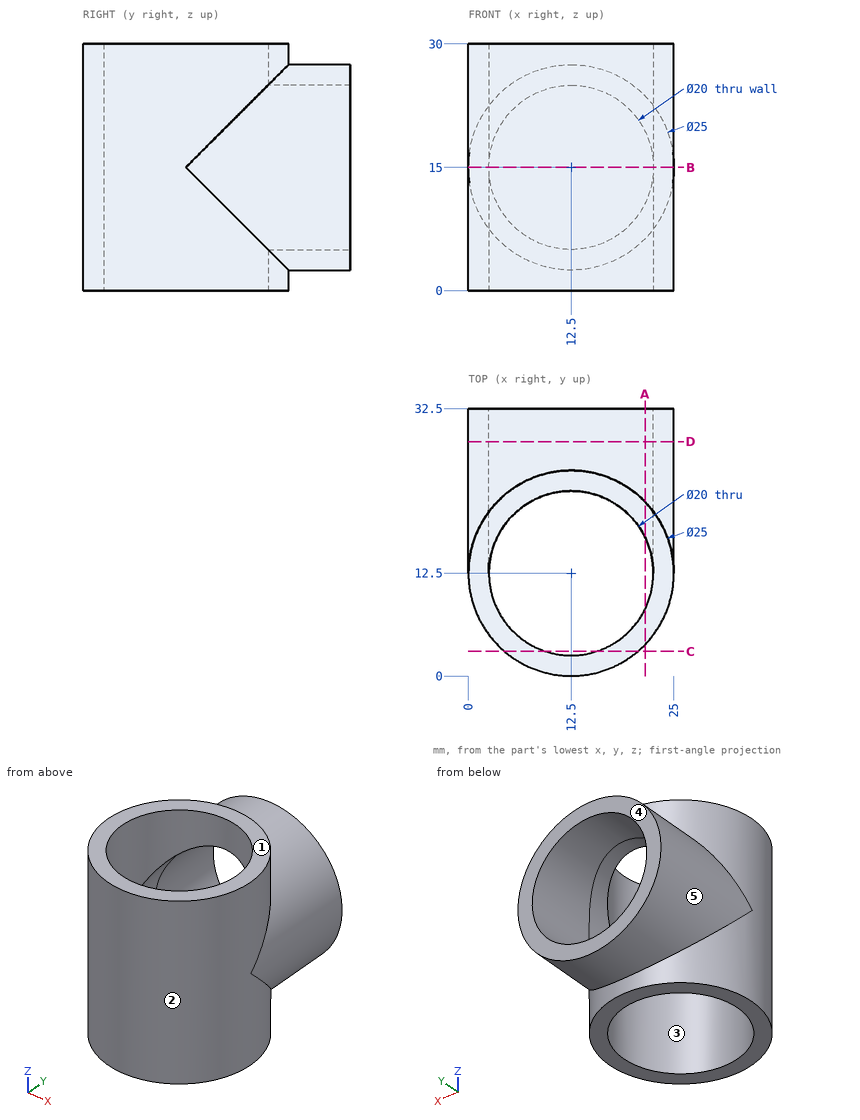
Study the drawing (mm; zero at the part's minimum x, y, z) and answer. A direction names the side the tool comes from. Give positions to 0.01 mm unless a question says otherwise; leave off trailing zeros. Loops run counter-clockwise (first coordinate to the right, second up) from the corner with the lowest first, then second, coordinate; pieces in that order, holes last. Notation, with made-up numbers: M 76.5,13.25 L 85.5,13.25 A28 ccw 85.5,38.25 Z; hole C -7,4 d9. An arc over 180 degrees is marked long. One line per item, written item: value.
1. Section D-D on y = 28.5 is taken. Determine the outline of the cut face in (x, z), plus the area to 3 significant figures.
Found:
outline: C 12.5,15 d25; hole C 12.5,15 d20
area: 177 mm^2
2. Find the intervals of material crossed by probe 1 along X at (y, z) = (12.5, 6.5); probe 2 along Y at (x, z) = (20.25, 5); probe 3 along X at (y, z) = (6, 18), in increasing order.
Found:
probe 1: 0 to 2.5, 22.5 to 25
probe 2: 2.69 to 6.18, 18.82 to 22.31
probe 3: 1.82 to 4.9, 20.1 to 23.18
3. Section B-B on z = 15 is taken. Determine the outline of the cut face in (x, y), plus the area to 3 significant figures.
Found:
outline: M 0,12.5 A12.5 ccw 25,12.5 L 25,32.5 L 22.5,32.5 L 22.5,12.5 A10 cw 2.5,12.5 L 2.5,32.5 L 0,32.5 Z
area: 188 mm^2
4. Section C-C on y = 3 is taken. Determine the outline of the cut face in (x, z), plus the area to 3 significant figures.
Found:
outline: M 4.38,0 L 9.38,0 L 9.38,30 L 4.38,30 Z; M 15.62,0 L 20.62,0 L 20.62,30 L 15.62,30 Z
area: 300 mm^2
5. Each of these flat-tipped pins is pushed along its axis until it touches: P1, Ø5, axis at y = 17, z = 19.5, coming from the +X side; P2, Ø2, axis at x = 13.5, z = 15.5, coming from the -Y side; P3, Ø1, axis at x = 17.5, z = 21, coming from the +Y side; P4, Ø12, axis at x = 12.5, y = 12.5, coming from the +Z side. Where does it stop, or does it pass through?
Found:
P1: x = 24.84
P2: y = 0
P3: y = 4.15
P4: through
6. For a pull along Y with two mould halves and no side action, classify the marked faces 1, 2 and 3 as pulls with the +Y half, pulls with the -Y half, needs draft (parallel to the pull), parting line crosses it, or undercut.
Found:
face 1: needs draft
face 2: parting line crosses it
face 3: undercut
7. Section A-A on x = 21.5 is taken. Determine the outline of the cut face in (y, z), plus the area to 3 significant figures.
Found:
outline: M 3.83,0 L 8.14,0 L 8.14,30 L 3.83,30 Z; M 16.86,0 L 21.17,0 L 21.17,6.33 L 32.5,6.33 L 32.5,10.64 L 16.86,10.64 Z; M 16.86,19.36 L 32.5,19.36 L 32.5,23.67 L 21.17,23.67 L 21.17,30 L 16.86,30 Z
area: 319 mm^2
8. For the marked faces 4 and 5, determine the directions among +Z, -Z, +X, -X, +Y, -Y from which every point of the face is accessible in a straight line to the end or side of a thin tool.
Found:
face 4: +Z, -Z, +X, -X, +Y
face 5: +Y
